For this review, use the dimensioned drawing (mm, ordinates from the lowest corner) and the shaded views. Give positions to 0.01 mm unless a question says otherwise; leave off trailing zeros. Write each loop counter-clockwise with the first axis right and the second up, starting at its lowest first coordinate (ties: lowest second). Pieces come first, ordered by that corner, then holes. Notation, with made-up numbers: (35, -10) -> (62, -10) arc R16 cw to (62, 20) -> close; hole circle Ø9 at (63, -37.5). An arc over 180 degrees is marked (long way). Answer as CSV lines item,"result".
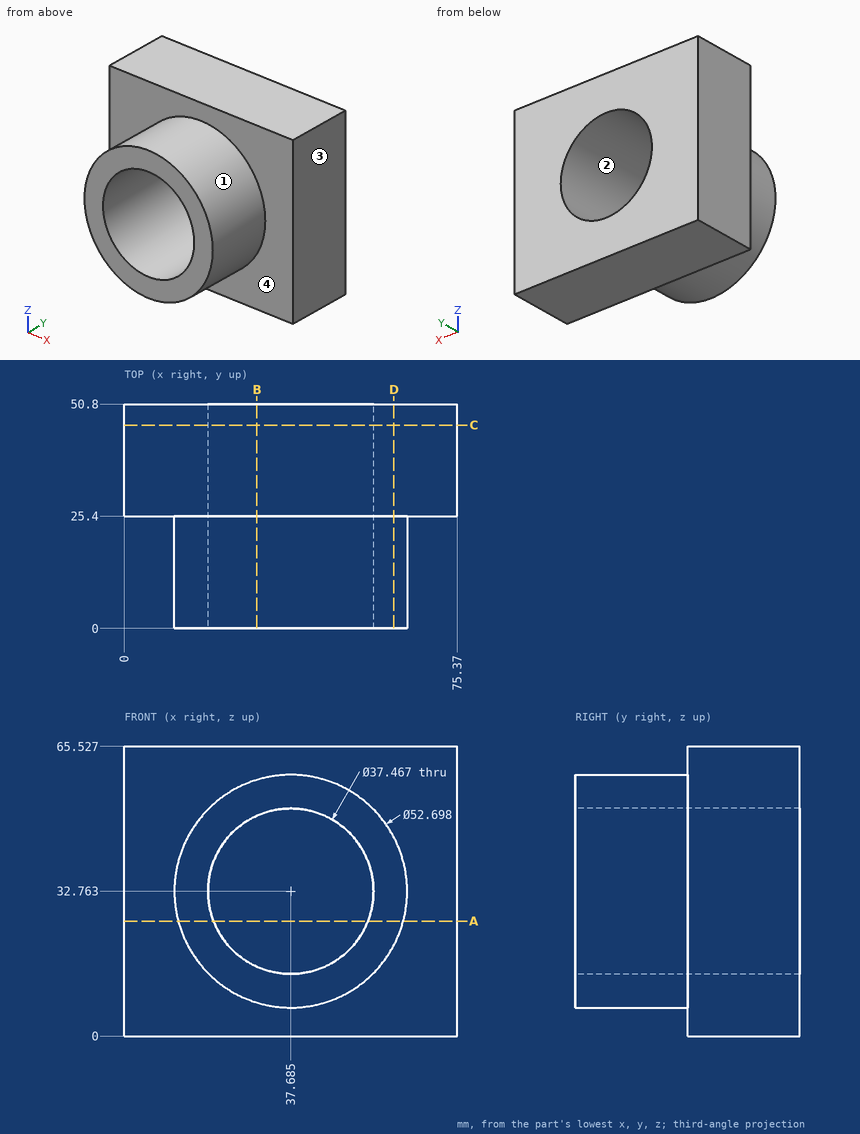
Q1. Add section B-B (x = 30). Write out the cut boundary in (y, z).
Answer block:
outline,"(0, 7.56) -> (25.4, 7.56) -> (25.4, 0) -> (50.8, 0) -> (50.8, 15.68) -> (0, 15.68) -> close; (0, 49.85) -> (50.8, 49.85) -> (50.8, 65.53) -> (25.4, 65.53) -> (25.4, 57.97) -> (0, 57.97) -> close"
Q2. Add section A-A (z = 26). Write out the cut boundary in (x, y) (1 decimal).
Answer block:
outline,"(0, 25.4) -> (12.2, 25.4) -> (12.2, 0) -> (20.2, 0) -> (20.2, 50.8) -> (0, 50.8) -> close; (55.2, 0) -> (63.2, 0) -> (63.2, 25.4) -> (75.4, 25.4) -> (75.4, 50.8) -> (55.2, 50.8) -> close"
Q3. Clearance check with flat-ended pins moving along their axes: pin 1 (4 mm diameter, centred on y = 33.5, z = 21.5, fed in from -X); pin 2 (5 mm diameter, centred on x = 45.5, y = 8, fed in from -Z); pin 3 (1 mm diameter, centred on x = 24.5, y = 15.5, fed in from +Z). State where each tip first meets the part, or that it passes through.
Answer block:
pin 1,"stops at x = 0"
pin 2,"stops at z = 6.96"
pin 3,"stops at z = 55.86"
Q4. Add section C-C (y = 46). Write out the cut boundary in (x, z) (1 decimal).
Answer block:
outline,"(0, 0) -> (75.4, 0) -> (75.4, 65.5) -> (0, 65.5) -> close; hole circle Ø37.5 at (37.7, 32.8)"
Q5. To check wall thickness, follow probe 1 along X at (y, z) = (35.5, 33.5); probe 2 along Y at (x, z) = (36, 3); probe 3 along X at (y, z) = (20.5, 18) (1 decimal). State the ranges of each line that lie inside material, in increasing order. Write a range as [from, to].
Answer block:
probe 1,"x = [0, 18.97], [56.4, 75.37]"
probe 2,"y = [25.4, 50.8]"
probe 3,"x = [15.9, 26.2], [49.2, 59.5]"
Q6. Add section D-D (x = 61). Write out the cut boundary in (y, z), plus the area to 3 significant figures.
Answer block:
outline,"(0, 20.49) -> (25.4, 20.49) -> (25.4, 0) -> (50.8, 0) -> (50.8, 65.53) -> (25.4, 65.53) -> (25.4, 45.04) -> (0, 45.04) -> close"
area,"2,290 mm2"
Q7. Draft analysis for pull direction X (two halves, no side actions). For the marked faces 1, 2, 3 and 4, state which applies: released by +X, released by -X, zero draft, split by the parting line, or undercut.
Answer block:
face 1,"split by the parting line"
face 2,"undercut"
face 3,"released by +X"
face 4,"zero draft"
